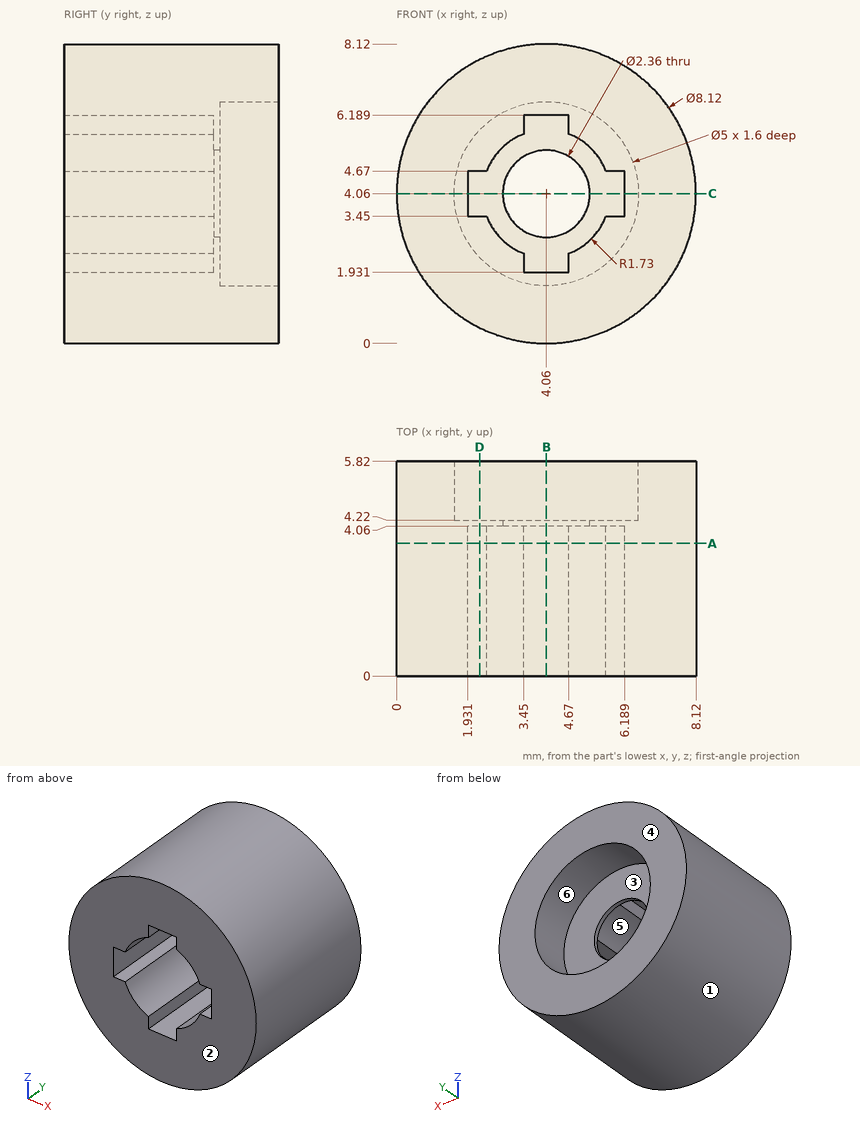
Input: dimensioned drawing with shaded views. Units: mm. Origin: part minimum x, y, z. A direction names the side the tool comes from. Coordinates: 2 decimals unless noted, no trailing zeros. Loops run counter-clockwise (first coordinate to the right, second up) from the corner with the lowest first, then second, coordinate; pieces in that order, holes last. Notation, with made-up numbers: M -2,86 L 49,86 A22 ccw 49,110 Z; hole C 80,82 d6. An arc over 180 degrees is marked long. Use a Markdown table: item, result. Add a question column.
Q1. Draft query along X for the marked faces 1, 2 and 3. Return one class per face: pulls with the +X half, pulls with the -X half, needs draft (parallel to the pull), parting line crosses it, or undercut.
Q2. Access query for the marked faces 4, 5 and 6. Directions: +Z, -Z, +X, -X, +Y, -Y. A direction counts if a zero-diameter tool reaches every point of the face in a straight line with its end or side. Return the directions, or none.
Q3. First-contact query: pin 1 (1.5 mm diameter, centred on y = 5, z = 2, fed in from -X); pin 2 (2 mm diameter, centred on x = 4.06, z = 4.06, fed in from -Y); pin 3 (1.5 mm diameter, centred on y = 1.5, z = 7, fed in from -X); pin 4 (1.5 mm diameter, centred on x = 5.5, y = 3.5, fed in from +Z). Flat tips, straight axial feed; report the tip coordinate or a pass-through.
Q4. Section query C-C, the plane z = 4.06. Return loops of the section in (x, y), and give its area (3 significant figures).
Q5. Material intervals for L1, parallel to X at y = 1.6, z = 4; L2, parallel to Z at x = 4.06, y = 4.9; L3, parallel to Z at x = 4.06, y = 4.15, sorted ascending.
Q6. Section query B-B, the plane x = 4.06. Return loops of the section in (y, z), and give its area (3 significant figures).
Q7. Section query D-D, the plane x = 2.25. Return loops of the section in (y, z).
Q8. Section query A-A, the plane y = 3.6. Return loops of the section in (x, z).
Result:
| question | item | result |
|---|---|---|
| 1 | face 1 | parting line crosses it |
| 1 | face 2 | needs draft |
| 1 | face 3 | undercut |
| 2 | face 4 | +Z, -Z, +X, -X, +Y |
| 2 | face 5 | -Y |
| 2 | face 6 | +Y |
| 3 | pin 1 | stops at x = 0.22 |
| 3 | pin 2 | passes through |
| 3 | pin 3 | stops at x = 0.64 |
| 3 | pin 4 | stops at z = 8.06 |
| 4 | outline | M 0,0 L 1.93,0 L 1.93,4.06 L 2.88,4.06 L 2.88,4.22 L 1.56,4.22 L 1.56,5.82 L 0,5.82 Z; M 5.24,4.06 L 6.19,4.06 L 6.19,0 L 8.12,0 L 8.12,5.82 L 6.56,5.82 L 6.56,4.22 L 5.24,4.22 Z |
| 4 | area | 21.6 mm2 |
| 5 | L1 | x = 0 to 1.93, 6.19 to 8.12 |
| 5 | L2 | z = 0 to 1.56, 6.56 to 8.12 |
| 5 | L3 | z = 0 to 2.88, 5.24 to 8.12 |
| 6 | outline | M 0,0 L 5.82,0 L 5.82,1.56 L 4.22,1.56 L 4.22,2.88 L 4.06,2.88 L 4.06,1.93 L 0,1.93 Z; M 0,6.19 L 4.06,6.19 L 4.06,5.24 L 4.22,5.24 L 4.22,6.56 L 5.82,6.56 L 5.82,8.12 L 0,8.12 Z |
| 6 | area | 21.6 mm2 |
| 7 | outline | M 0,0.43 L 5.82,0.43 L 5.82,2.34 L 4.22,2.34 L 4.22,5.78 L 5.82,5.78 L 5.82,7.69 L 0,7.69 L 0,4.67 L 4.06,4.67 L 4.06,3.45 L 0,3.45 Z |
| 8 | outline | C 4.06,4.06 d8.12; hole M 1.93,3.45 L 2.44,3.45 A1.73 ccw 3.45,2.44 L 3.45,1.93 L 4.67,1.93 L 4.67,2.44 A1.73 ccw 5.68,3.45 L 6.19,3.45 L 6.19,4.67 L 5.68,4.67 A1.73 ccw 4.67,5.68 L 4.67,6.19 L 3.45,6.19 L 3.45,5.68 A1.73 ccw 2.44,4.67 L 1.93,4.67 Z |
